from build123d import *

# Parameters (mm, degrees)
SKETCH1_W             = 12
SKETCH1_H             = 19
BOSS_EXTRUDE1_DEPTH   = 11
SKETCH2_W             = 15
SKETCH2_H             = 21
SKETCH2_W_2           = 10
SKETCH2_H_2           = 16
BOSS_EXTRUDE2_DEPTH   = 2
CHAMFER1_SIZE         = 1
CHAMFER1_SIZE2        = 1.732050808
CHAMFER1_PART_2_SIZE  = 1
CHAMFER1_PART_2_SIZE2 = 1.732050808
CHAMFER1_PART_3_SIZE  = 1
CHAMFER1_PART_3_SIZE2 = 1.732050808
CHAMFER1_PART_4_SIZE  = 1
CHAMFER1_PART_4_SIZE2 = 1.732050808
BOSS_EXTRUDE3_DEPTH   = 10
SKETCH4_W             = 4.8
SKETCH4_H             = 0.6
BOSS_EXTRUDE4_DEPTH   = 8


with BuildPart() as part:
    # Sketch1 → Boss-Extrude1 (new body)
    with BuildSketch(Plane(origin=(0, 0, 0), x_dir=(1, 0, 0), z_dir=(0, 1, 0))):
        Rectangle(SKETCH1_W, SKETCH1_H)
    extrude(amount=BOSS_EXTRUDE1_DEPTH)

    # Sketch2 → Boss-Extrude2 (add)
    with BuildSketch(Plane(origin=(0, 11, 0), x_dir=(1, 0, 0), z_dir=(0, 1, 0))):
        Rectangle(SKETCH2_W, SKETCH2_H)
        Rectangle(SKETCH2_W_2, SKETCH2_H_2, mode=Mode.SUBTRACT)
    extrude(amount=BOSS_EXTRUDE2_DEPTH)

    # Chamfer1
    chamfer1_edges = [part.edges().sort_by_distance(p)[0] for p in [
        (-7.5, 13, 0),
    ]]
    chamfer1_side = [part.faces().sort_by_distance(p)[0] for p in [
        (-7.5, 12, 0),
    ]]
    chamfer(chamfer1_edges, length=CHAMFER1_SIZE, length2=CHAMFER1_SIZE2, reference=chamfer1_side[0])

    # Chamfer1 part 2
    chamfer1_part_2_edges = [part.edges().sort_by_distance(p)[0] for p in [
        (0, 13, 10.5),
    ]]
    chamfer1_part_2_side = [part.faces().sort_by_distance(p)[0] for p in [
        (0, 12, 10.5),
    ]]
    chamfer(chamfer1_part_2_edges, length=CHAMFER1_PART_2_SIZE, length2=CHAMFER1_PART_2_SIZE2, reference=chamfer1_part_2_side[0])

    # Chamfer1 part 3
    chamfer1_part_3_edges = [part.edges().sort_by_distance(p)[0] for p in [
        (7.5, 13, 0),
    ]]
    chamfer1_part_3_side = [part.faces().sort_by_distance(p)[0] for p in [
        (7.5, 12, 0),
    ]]
    chamfer(chamfer1_part_3_edges, length=CHAMFER1_PART_3_SIZE, length2=CHAMFER1_PART_3_SIZE2, reference=chamfer1_part_3_side[0])

    # Chamfer1 part 4
    chamfer1_part_4_edges = [part.edges().sort_by_distance(p)[0] for p in [
        (0, 13, -10.5),
    ]]
    chamfer1_part_4_side = [part.faces().sort_by_distance(p)[0] for p in [
        (0, 12, -10.5),
    ]]
    chamfer(chamfer1_part_4_edges, length=CHAMFER1_PART_4_SIZE, length2=CHAMFER1_PART_4_SIZE2, reference=chamfer1_part_4_side[0])

    # Sketch3 → Boss-Extrude3 (add)
    with BuildSketch(Plane(origin=(-5, 0, 0), x_dir=(0, 0, -1), z_dir=(1, 0, 0))):
        with BuildLine():
            Line((-8.767949192, 13), (-8.767949192, 12))
            Line((-8.767949192, 12), (9.162687499, 12))
            ThreePointArc((9.162687499, 12), (7.670106688, 15.172024144), (5.622167077, 18.017279493))
            ThreePointArc((5.622167077, 18.017279493), (-1.14809782, 14.290285439), (-8.767949192, 13))
        make_face()
    extrude(amount=BOSS_EXTRUDE3_DEPTH)

    # Sketch4 → Boss-Extrude4 (add)
    with BuildSketch(Plane.XZ):
        with Locations((0, -7.2)):
            Rectangle(SKETCH4_W, SKETCH4_H)
        with Locations((0, -0.04)):
            Rectangle(SKETCH4_W, SKETCH4_H)
    extrude(amount=BOSS_EXTRUDE4_DEPTH)


solid = part.part
Design review of the part built by this model. Coordinates are the model's own, in mm. A direction names the side the tool comes from. Give positions to 0.01 mm unless a question says otherwise; leave off trailing zeros. Loops run counter-clockwise (first coordinate to the right, second up) from the corner with the lowest first, then second, coordinate; pieces in that order, holes last. Notation, with made-up numbers: M -31,44 L -19,44 A23 ccw -19,67 Z; hole C 80,10.25 d10. An arc over 180 degrees is marked long. One line per question, with ' | ' between items. Start each with the question number.
1. Add section C-C (z = -6). Write out the cut boundary in (x, y).
2. Add section B-B (x = 3). Write out the cut boundary in (y, z).
3. Add section D-D (x = -0.5). Write out the cut boundary in (y, z), plus the area to 3 significant figures.
4. To check wall thickness, follow L1, parallel to Z at x = 1, y = -4.75; L2, parallel to Z at x = 0.25, y = 3; L3, parallel to X at y = 15, z = -3.25. State the ranges of each line that lie inside material, in increasing order.
5. For faces 1 (the face through (0, -4, -0.34)), 2 (the face through (-6, 5, 0)), 3 (the face through (0, 5, 9.5)), list the 3-axis set-ups (+Z, -Z, +X, -X, +Y, -Y) from which the entire face can be reached by the end or side of a thin tool; tool diameter is ignored.
6. The part is to be moulded in two halves that separate along Y. For faces 4 (the face through (-0.07, 14.326, 1.046)), 5 (the face through (5, 14, -4)), 6 (the face through (-0.1, 11.5, -8)), 7 (the face through (0, 11, 0)), say which applies: released by +Y, released by -Y, zero draft, split by the parting line, or undercut.
7. Add section A-A (y = -6.25). Write out the cut boundary in (x, z), plus the area to 3 significant figures.
8. Insertion check: P1, Ø2, axis at x = -1, z = -7, coming from the +Y side; P2, Ø2, axis at x = 2, y = 8, coming from the -Z side; P3, Ø4, axis at y = 15.5, z = 1, coming from the +X side. Each pin has a flat end and moves straight along its axis. Give the tip position at first contact, or say it passes through.
Worked out:
1) outline: M -7.5,11 L -6,11 L -6,0 L 6,0 L 6,11 L 7.5,11 L 7.5,12 L 5.77,13 L 5,13 L 5,17.57 L -5,17.57 L -5,13 L -5.77,13 L -7.5,12 Z; hole M -5,11 L 5,11 L 5,12 L -5,12 Z
2) outline: M 0,-9.5 L 11,-9.5 L 11,-10.5 L 12,-10.5 L 13,-8.77 A19.07 ccw 18.02,-5.62 A23.14 cw 13,8.77 L 12,10.5 L 11,10.5 L 11,9.5 L 0,9.5 Z; hole M 11,-8 L 12,-8 L 12,8 L 11,8 Z
3) outline: M -8,-7.5 L 0,-7.5 L 0,-9.5 L 11,-9.5 L 11,-10.5 L 12,-10.5 L 13,-8.77 A19.07 ccw 18.02,-5.62 A23.14 cw 13,8.77 L 12,10.5 L 11,10.5 L 11,9.5 L 0,9.5 L 0,0.26 L -8,0.26 L -8,-0.34 L 0,-0.34 L 0,-6.9 L -8,-6.9 Z; hole M 11,-8 L 12,-8 L 12,8 L 11,8 Z | area: 275 mm²
4) L1: z = -7.5 to -6.9, -0.34 to 0.26 | L2: z = -9.5 to 9.5 | L3: x = -5 to 5
5) face 1: +X, -X, -Y | face 2: +Z, -Z, -X, -Y | face 3: +Z, +X, -X, -Y
6) face 4: released by +Y | face 5: zero draft | face 6: undercut | face 7: undercut
7) outline: M -2.4,-7.5 L 2.4,-7.5 L 2.4,-6.9 L -2.4,-6.9 Z; M -2.4,-0.34 L 2.4,-0.34 L 2.4,0.26 L -2.4,0.26 Z | area: 5.76 mm²
8) P1: stops at y = 17.57 | P2: stops at z = -9.5 | P3: stops at x = 5
